from build123d import *

# Parameters (mm, degrees)
SKETCH1_R           = 12.7
BOSS_EXTRUDE1_DEPTH = 12.7
SKETCH2_R           = 15.24
BOSS_EXTRUDE2_DEPTH = 5


with BuildPart() as part:
    # Sketch1 → Boss-Extrude1 (new body, symmetric)
    with BuildSketch(Plane(origin=(0, 0, 0), x_dir=(1, 0, 0), z_dir=(0, 1, 0))):
        Circle(SKETCH1_R)
    extrude(amount=BOSS_EXTRUDE1_DEPTH, both=True)

    # Sketch2 → Boss-Extrude2 (add)
    with BuildSketch(Plane(origin=(0, 12.7, 0), x_dir=(1, 0, 0), z_dir=(0, 1, 0))):
        Circle(SKETCH2_R)
    boss_extrude2 = extrude(amount=BOSS_EXTRUDE2_DEPTH)

    # Mirror1: Boss-Extrude2 across plane
    add(boss_extrude2.mirror(Plane.ZX))


solid = part.part
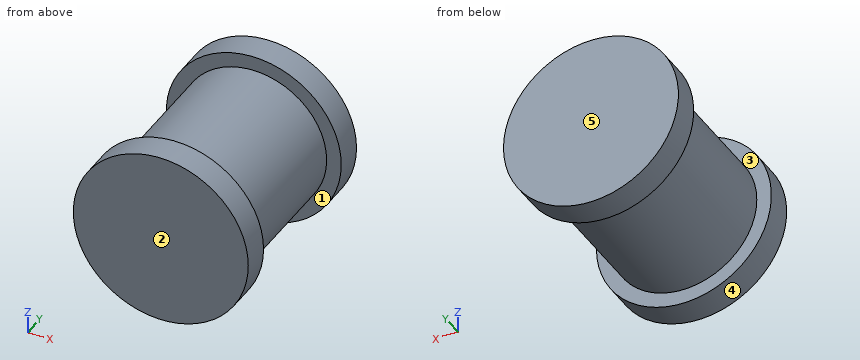
Can you work these out from the model? Positions are in its coordinate system, mm. Face numbers are marked on the shaded views. A direction names the side the tool comes from. Coordinates: 2 decimals unless noted, no trailing zeros. Write each loop counter-clockwise with the first axis right and the second up, starting at its lowest first coordinate (ties: lowest second). Pieces come first, ordered by that corner, then holes. Notation, with made-up numbers: (64.25, 32.5) -> (100.25, 32.5) arc R22 ccw to (100.25, 56.5) -> close; hole circle Ø1 at (11.5, 9.5). An arc over 180 degrees is marked (long way). Write each question's results on one line, items separated by ' | '. Start each with the question number.
Item 1: If we section it at A-A, the plane x = 0: Write out the boundary of the cut face in (y, z).
Item 2: I'm going to push flat-ended pins straight in: P1, Ø1.5, axis at y = 5, z = 1.5, coming from the +X side; P2, Ø6, axis at y = -13, z = -6.5, coming from the -X side; P3, Ø4, axis at y = -6.5, z = -7.5, coming from the +X side. Where does each tip first touch, or does it pass through?
Item 3: On a 3-axis mill with a long thin cutter (end or side, diameter ignored), from which of +Z, -Z, +X, -X, +Y, -Y can I reach the whole of each face in a straight line? I mean the marked faces 1 and 2. Say none if no direction works.
Item 4: If we section it at B-B, the plane z = 0: Write out the boundary of the cut face in (x, y).
Item 5: If we section it at C-C, the plane y = 10: Write out the boundary of the cut face in (x, z).
Item 6: Thinking about a two-plate mould opening in Y: for the marked faces 3, 4 and 5, which applies, released by +Y, released by -Y, zero draft, split by the parting line, or undercut?
Item 7: Please list where these lines run through material, in increasing order: probe 1 along Y at (x, z) = (-0.5, 13); probe 2 along Z at (x, y) = (-0.5, 3.5); probe 3 along X at (y, z) = (-1, 6.5).
Answer block:
1) outline: (-17.7, -15.24) -> (-12.7, -15.24) -> (-12.7, -12.7) -> (12.7, -12.7) -> (12.7, -15.24) -> (17.7, -15.24) -> (17.7, 15.24) -> (12.7, 15.24) -> (12.7, 12.7) -> (-12.7, 12.7) -> (-12.7, 15.24) -> (-17.7, 15.24) -> close
2) P1: x = 12.68 | P2: x = -14.83 | P3: x = 11.45
3) face 1: none | face 2: +Z, -Z, +X, -X, -Y
4) outline: (-15.24, -17.7) -> (15.24, -17.7) -> (15.24, -12.7) -> (12.7, -12.7) -> (12.7, 12.7) -> (15.24, 12.7) -> (15.24, 17.7) -> (-15.24, 17.7) -> (-15.24, 12.7) -> (-12.7, 12.7) -> (-12.7, -12.7) -> (-15.24, -12.7) -> close
5) outline: circle Ø25.4 at (0, 0)
6) face 3: undercut | face 4: zero draft | face 5: released by +Y
7) probe 1: -17.7 to -12.7, 12.7 to 17.7 | probe 2: -12.69 to 12.69 | probe 3: -10.91 to 10.91
